The model under review builds one solid part; all positions refer to its coordinate system, in mm. A direction names the side the tool comes from. Round coordinates to 2 decimals unless told otherwise and drop trailing zeros. Write each loop counter-clockwise with the first axis right and the second up, starting at its lowest first coordinate (ties: lowest second). Pieces come first, ordered by that corner, then holes.
Item 1: Clearance check with flat-ended pins moving along their axes: pin 1 Ø3.5 at (y, z) = (-2, 1.5) entering from +X; pin 2 Ø0.9 at (x, y) = (-1.5, 82) entering from +Z; pin 3 Ø12 at (y, z) = (17.5, -17) entering from +X. State where each tip first meets the part, or that it passes through.
Item 2: Add section A-A (x = 39.5). Give the boundary of the cut face in (y, z).
Item 3: Add section C-C (z = -13). Give the boundary of the cut face in (x, y).
Item 4: To check wall thickness, follow L1, parallel to X at y = 5.5, z = 0; L2, parallel to X at y = 2.75, z = 0; L3, parallel to Z at x = 33.5, y = 3. State the ranges of each line that lie inside material, in increasing order.
Item 5: Machinability: for faces 1 (the face through (7, 46, -6)), 2 (the face through (6, -1, 0)), 3 (the face through (3.55, 15.75, 0.09)), 4 (the face through (83, -1, 0)), 5 (the face through (-1, 81, 5)), which of the approach directions +Z, -Z, +X, -X, +Y, -Y give a long, thin tool a straight path to every point of the face, cutting with its end or side? Answer none if there is none.
Item 6: Draft analysis for pull direction Z (two halves, no side actions). For faces 6 (the face through (4, 33, -4.25)), 7 (the face through (34, 34, 21.5)), 8 (the face through (42, 0, 5)), 9 (the face through (3.55, 50.25, -0.09)), state which applies: +Z half, -Z half, draft (parallel to the pull), parting line (faces both ways), or undercut.
Item 7: Add section B-B (y = 68). Give the boundary of the cut face in (x, z), plus the area to 4 significant figures.
Item 8: Add section D-D (x = 52). Give the boundary of the cut face in (y, z), plus the area to 3 significant figures.
```python
from build123d import *

# Parameters (mm, degrees)
EXTRUDE_1_DEPTH     = 21.5
EXTRUDE_2_DEPTH     = 4
SKETCH_3_R          = 4.25
CUT_EXTRUDE_1_DEPTH = 8
SKETCH_4_W          = 3
SKETCH_4_H          = 10
EXTRUDE_3_DEPTH     = 3


with BuildPart() as part:
    # Эскиз1 → Бобышка-Вытянуть1 (new body, symmetric)
    with BuildSketch(Plane.XY):
        Polygon((0, 86), (0, 0), (86, 0), (86, 7), (7, 7), (7, 86), align=None)
    extrude(amount=EXTRUDE_1_DEPTH, both=True)

    # Эскиз2 → Бобышка-Вытянуть2 (add)
    with BuildSketch(Plane.XY.offset(21.5)):
        Polygon((86, 7), (7, 7), (7, 86), (14, 86), (86, 14), align=None)
    extrude(amount=-EXTRUDE_2_DEPTH)

    # Эскиз3 → Вырез-Вытянуть1 (cut, through all)
    with BuildSketch(Plane(origin=(0, 7, 0), x_dir=(1, 0, 0), z_dir=(0, 1, 0))):
        with Locations(Location((68, 0, 0), (0, 0, 270))):  # turned: the seam where the file's is
            Circle(SKETCH_3_R)
        with BuildLine():
            Line((20, 4.25), (46, 4.25))
            ThreePointArc((46, 4.25), (50.25, 0), (46, -4.25))
            Line((46, -4.25), (20, -4.25))
            ThreePointArc((20, -4.25), (15.75, 0), (20, 4.25))
        make_face()
    cut_extrude_1 = extrude(amount=-CUT_EXTRUDE_1_DEPTH, mode=Mode.SUBTRACT)

    # Эскиз4 → Бобышка-Вытянуть3 (add)
    with BuildSketch(Plane.XZ):
        with Locations((4.5, 0)):
            Rectangle(SKETCH_4_W, SKETCH_4_H)
        with Locations((81.5, 0)):
            Rectangle(SKETCH_4_W, SKETCH_4_H)
    extrude_3 = extrude(amount=EXTRUDE_3_DEPTH)

    # Зеркальное отражение3: Вырез-Вытянуть1, Бобышка-Вытянуть3 across plane
    add(cut_extrude_1.mirror(Plane(origin=(0, 0, 0), x_dir=(0, 0, 1), z_dir=(-0.707106781, 0.707106781, 0))), mode=Mode.SUBTRACT)
    add(extrude_3.mirror(Plane(origin=(0, 0, 0), x_dir=(0, 0, 1), z_dir=(-0.707106781, 0.707106781, 0))))


solid = part.part
```
Numbers:
1. pin 1: stops at x = 83
1. pin 2: stops at z = 5
1. pin 3: stops at x = 7
2. outline: (0, -21.5) - (7, -21.5) - (7, -4.25) - (0, -4.25) - close; (0, 4.25) - (7, 4.25) - (7, 17.5) - (60.5, 17.5) - (60.5, 21.5) - (0, 21.5) - close
3. outline: (0, 0) - (86, 0) - (86, 7) - (7, 7) - (7, 86) - (0, 86) - close
4. L1: x = -3 to 15.75, 50.25 to 63.75, 72.25 to 86
4. L2: x = 0 to 15.75, 50.25 to 63.75, 72.25 to 86
4. L3: z = -21.5 to -4.25, 4.25 to 21.5
5. face 1: -Z, +X, +Y
5. face 2: +Z, -Z, -Y
5. face 3: +X, -X
5. face 4: +Z, -Z, +X, -Y
5. face 5: +Z, -X, +Y, -Y
6. face 6: undercut
6. face 7: +Z half
6. face 8: draft
6. face 9: undercut
7. outline: (0, -21.5) - (7, -21.5) - (7, -4.25) - (0, -4.25) - close; (0, 4.25) - (7, 4.25) - (7, 17.5) - (32, 17.5) - (32, 21.5) - (0, 21.5) - close
7. area: 341.5 mm2
8. outline: (0, -21.5) - (7, -21.5) - (7, 17.5) - (48, 17.5) - (48, 21.5) - (0, 21.5) - close
8. area: 465 mm2
